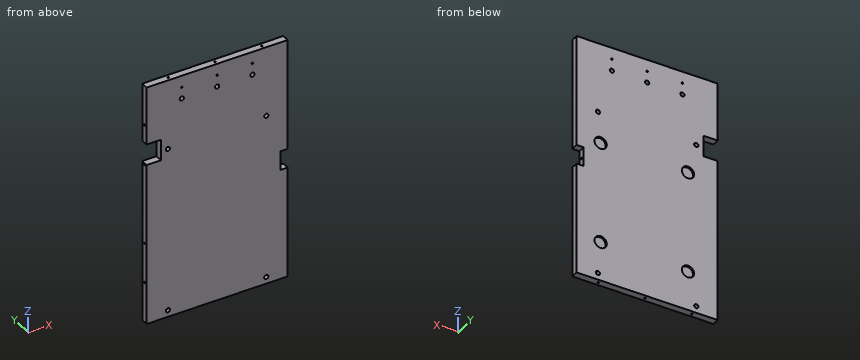
```python
from build123d import *

# Parameters (mm, degrees)
SKETCH_1_W          = 59.5
SKETCH_1_H          = 103.8
EXTRUDE_1_DEPTH     = 3
SKETCH_2_R          = 2.6
CUT_EXTRUDE_1_DEPTH = 0.8
SKETCH_3_W          = 8.2
SKETCH_3_H          = 3
CUT_EXTRUDE_2_DEPTH = 3
CUT_EXTRUDE_START   = -3
SKETCH_3_3_R        = 0.35
CUT_EXTRUDE_4_DEPTH = 3
SKETCH_4_R          = 0.35
CUT_EXTRUDE_5_DEPTH = 3
SKETCH_5_R          = 0.35
CUT_EXTRUDE_6_DEPTH = 3
SKETCH_8_W          = 6
SKETCH_8_H          = 9
CUT_EXTRUDE_7_DEPTH = 60.897182738
SKETCH_9_R          = 0.9
CUT_EXTRUDE_8_DEPTH = 60.897182738
SKETCH_10_R         = 0.35
SKETCH_10_R_2       = 0.9
CUT_EXTRUDE_9_DEPTH = 60.89718283


with BuildPart() as part:
    # 草图1 → 凸台-拉伸1 (new body)
    with BuildSketch(Plane(origin=(0, 0, 0), x_dir=(1, 0, 0), z_dir=(0, 1, 0))):
        Rectangle(SKETCH_1_W, SKETCH_1_H)
    extrude(amount=EXTRUDE_1_DEPTH)

    # 草图2 → 切除-拉伸1 (cut)
    with BuildSketch(Plane(origin=(0, 3, 0), x_dir=(1, 0, 0), z_dir=(0, 1, 0))):
        with Locations(Location((19.612933951, 35, 0), (0, 0, 270))):
            Circle(SKETCH_2_R)
        with Locations(Location((19.612933951, -8.5, 0), (0, 0, 270))):
            Circle(SKETCH_2_R)
        with Locations(Location((-17.24, -8.5, 0), (0, 0, 270))):
            Circle(SKETCH_2_R)
        with Locations(Location((-17.24, 35, 0), (0, 0, 270))):
            Circle(SKETCH_2_R)
    extrude(amount=-CUT_EXTRUDE_1_DEPTH, mode=Mode.SUBTRACT)

    # 草图3 → 切除-拉伸2 (cut)
    with BuildSketch(Plane(origin=(29.75, 0, 0), x_dir=(0, 0, -1), z_dir=(1, 0, 0))):
        with Locations((0, 1.5)):
            Rectangle(SKETCH_3_W, SKETCH_3_H)
    extrude(amount=-CUT_EXTRUDE_2_DEPTH, mode=Mode.SUBTRACT)

    # 草图3<3> → 切除-拉伸4 (cut)
    with BuildSketch(Plane(origin=(29.75, 0, 0), x_dir=(0, 0, -1), z_dir=(1, 0, 0)).offset(CUT_EXTRUDE_START)):
        with Locations((0, 1.5)):
            Circle(SKETCH_3_3_R)
    extrude(amount=-CUT_EXTRUDE_4_DEPTH, mode=Mode.SUBTRACT)

    # 草图4 → 切除-拉伸5 (cut)
    with BuildSketch(Plane(origin=(0, 0, -51.9), x_dir=(-1, 0, 0), z_dir=(0, 0, -1))):
        with Locations((-19.75, 1.5)):
            Circle(SKETCH_4_R)
        with Locations((0, 1.5)):
            Circle(SKETCH_4_R)
        with Locations((19.75, 1.5)):
            Circle(SKETCH_4_R)
    cut_extrude_5 = extrude(amount=-CUT_EXTRUDE_5_DEPTH, mode=Mode.SUBTRACT)

    # 草图5 → 切除-拉伸6 (cut)
    with BuildSketch(Plane.ZY.offset(29.75)):
        with Locations((-34.6, 1.5)):
            Circle(SKETCH_5_R)
        with Locations((-17.3, 1.5)):
            Circle(SKETCH_5_R)
    cut_extrude_6 = extrude(amount=-CUT_EXTRUDE_6_DEPTH, mode=Mode.SUBTRACT)

    # 镜向1: 切除-拉伸5, 切除-拉伸6 across plane
    add(cut_extrude_5.mirror(Plane.XY), mode=Mode.SUBTRACT)
    add(cut_extrude_6.mirror(Plane.XY), mode=Mode.SUBTRACT)

    # 草图8 → 切除-拉伸7 (cut, through all)
    with BuildSketch(Plane(origin=(0, 3, 0), x_dir=(1, 0, 0), z_dir=(0, 1, 0))):
        with Locations((-26.75, -22.4)):
            Rectangle(SKETCH_8_W, SKETCH_8_H)
    extrude(amount=-CUT_EXTRUDE_7_DEPTH, mode=Mode.SUBTRACT)

    # 草图9 → 切除-拉伸8 (cut, through all)
    with BuildSketch(Plane(origin=(0, 3, 0), x_dir=(1, 0, 0), z_dir=(0, 1, 0))):
        with Locations(Location((-20.75, 49, 0), (0, 0, 270))):
            Circle(SKETCH_9_R)
        with Locations(Location((20.75, 49, 0), (0, 0, 270))):
            Circle(SKETCH_9_R)
        with Locations(Location((-20.75, -21.8, 0), (0, 0, 270))):
            Circle(SKETCH_9_R)
        with Locations(Location((20.75, -21.8, 0), (0, 0, 270))):
            Circle(SKETCH_9_R)
    extrude(amount=-CUT_EXTRUDE_8_DEPTH, mode=Mode.SUBTRACT)

    # 草图10 → 切除-拉伸9 (cut, through all)
    with BuildSketch(Plane(origin=(0, 3, 0), x_dir=(1, 0, 0), z_dir=(0, 1, 0))):
        with Locations(Location((14.875, -46.9, 0), (0, 0, 270))):
            Circle(SKETCH_10_R)
        with Locations(Location((-14.875, -46.9, 0), (0, 0, 270))):
            Circle(SKETCH_10_R)
        with Locations(Location((14.875, -41.9, 0), (0, 0, 270))):
            Circle(SKETCH_10_R_2)
        with Locations(Location((-14.875, -41.9, 0), (0, 0, 270))):
            Circle(SKETCH_10_R_2)
        with Locations(Location((0, -46.9, 0), (0, 0, 270))):
            Circle(SKETCH_10_R)
        with Locations(Location((0, -41.9, 0), (0, 0, 270))):
            Circle(SKETCH_10_R_2)
    extrude(amount=-CUT_EXTRUDE_9_DEPTH, mode=Mode.SUBTRACT)


solid = part.part
```
Work out the finished part from the listing and answer in its coordinate system (mm). Coordinates: 2 decimals unless noted, no trailing zeros. Order: outer loops, then holes, each group sorted by start corner. A loop starts at its lowest first (then second) coordinate and runs counter-clockwise, first axis right, second up. Notation, with made-up numbers: (34, 47.25) - (76, 47.25) arc R18 cw to (76, 70.25) - close; hole circle Ø1 at (31.5, 72). An arc over 180 degrees is marked (long way). Answer as a JSON object with one key per item and string values.
1. Find section A-A on z = 8.5. Determine the outline of the cut face in (x, y).
Output values:
{"outline": "(-29.75, 0) - (29.75, 0) - (29.75, 3) - (22.21, 3) - (22.21, 2.2) - (17.01, 2.2) - (17.01, 3) - (-14.64, 3) - (-14.64, 2.2) - (-19.84, 2.2) - (-19.84, 3) - (-29.75, 3) - close"}
2. Consider line 1 (X direction, y = 0.95, z = 46.9) (3 decimals); line 2 (X direction, y = 2.2, z = 41.9) (3 decimals); line 3 (Y direction, x = 19.75, z = -49.5). Determine where each line is inside the solid, lowest interval first.
Output values:
{"line 1": "x = -29.75 to -15.225, -14.525 to -0.35, 0.35 to 14.525, 15.225 to 29.75", "line 2": "x = -29.75 to -15.775, -13.975 to -0.9, 0.9 to 13.975, 15.775 to 29.75", "line 3": "y = 0 to 1.15, 1.85 to 3"}
3. Find section B-B on x = -17.24. Determine the outline of the cut face in (y, z).
Output values:
{"outline": "(0, -51.9) - (3, -51.9) - (3, -37.6) - (2.2, -37.6) - (2.2, -32.4) - (3, -32.4) - (3, 5.9) - (2.2, 5.9) - (2.2, 11.1) - (3, 11.1) - (3, 51.9) - (0, 51.9) - close"}
4. Find section C-C on z = 25.5. Determine the outline of the cut face in (x, y).
Output values:
{"outline": "(-23.75, 0) - (29.75, 0) - (29.75, 3) - (-23.75, 3) - close"}
5. Each of these flat-tipped pins is pushed along its axis until it touches: P1, Ø4.5, axis at x = -17.24, z = 8.5, coming from the -Y side; P2, Ø1.6, axis at x = 18.5, z = -34.5, coming from the +Y side. Where does it stop, or does it pass through?
Output values:
{"P1": "stops at y = 0", "P2": "stops at y = 2.2"}
